Answer from the drawing. Dimensions are ordinates in mm from the lowest x, y and z of the part. A direction names the side the tool comes from. Coordinates: 2 decimals unless noted, no trailing zeros. Order: outer loops, then holes, each group sorted by start corner. A loop starts at its lowest first (then second) coordinate and runs counter-clockwise, first axis right, second up. Notation, with made-up numbers: (54.25, 23) - (79.25, 23) arc R12 cw to (79.25, 43) - close; hole circle Ø2 at (60, 32). An arc over 180 degrees is marked (long way). Answer as a JSON object with one key per item and string values. Group by question number.
1) Section C-C (z = 80.5) is taken. Count the separate pieces of the cut face and the enclosed holes in it, plus the area to 3 significant figures.
2) The mould has two halves that part along X. Classify the marked faces 1, 2 and 3: released by +X, released by -X, zero draft, split by the parting line, or undercut.
3) A tool of negligible diameter and unlimited length cuts with its end or side. For the marked faces 4, 5, 6, 7 and 8, from which of +Z, -Z, +X, -X, +Y, -Y can it reach the whole face along a straight path? Write none if from no direction.
4) Each of these flat-tipped pins is pushed along its axis until it touches: P1, Ø5, axis at x = 74, y = 104.5, coming from the +Z side; P2, Ø5, axis at x = 54, z = 22.5, coming from the +Y side; P3, Ø2, axis at x = 63, z = 83.5, coming from the -Y side; P4, Ø12, axis at x = 94, z = 77.5, coming from the -Y side. Where does it stop, or does it pass through?
5) Section A-A (z = 15) is taken. Give the vertices of the cut face in (x, y) (1 decimal), plus the area to 3 significant figures.
6) Section B-B (y = 87) is taken. Give the vertices of the cut face in (x, z) (1 decimal), plus the area to 3 significant figures.
7) Section D-D (x = 64.5) is taken. Give the vertices of the cut face in (y, z) (1 decimal).
8) Find the intervals of material crossed by line 1 along Z through (x, y) = (31, 68); line 2 along X through (y, z) = (66, 74.5); line 3 along X through (y, z) = (38, 81) (1 decimal), in increasing order.
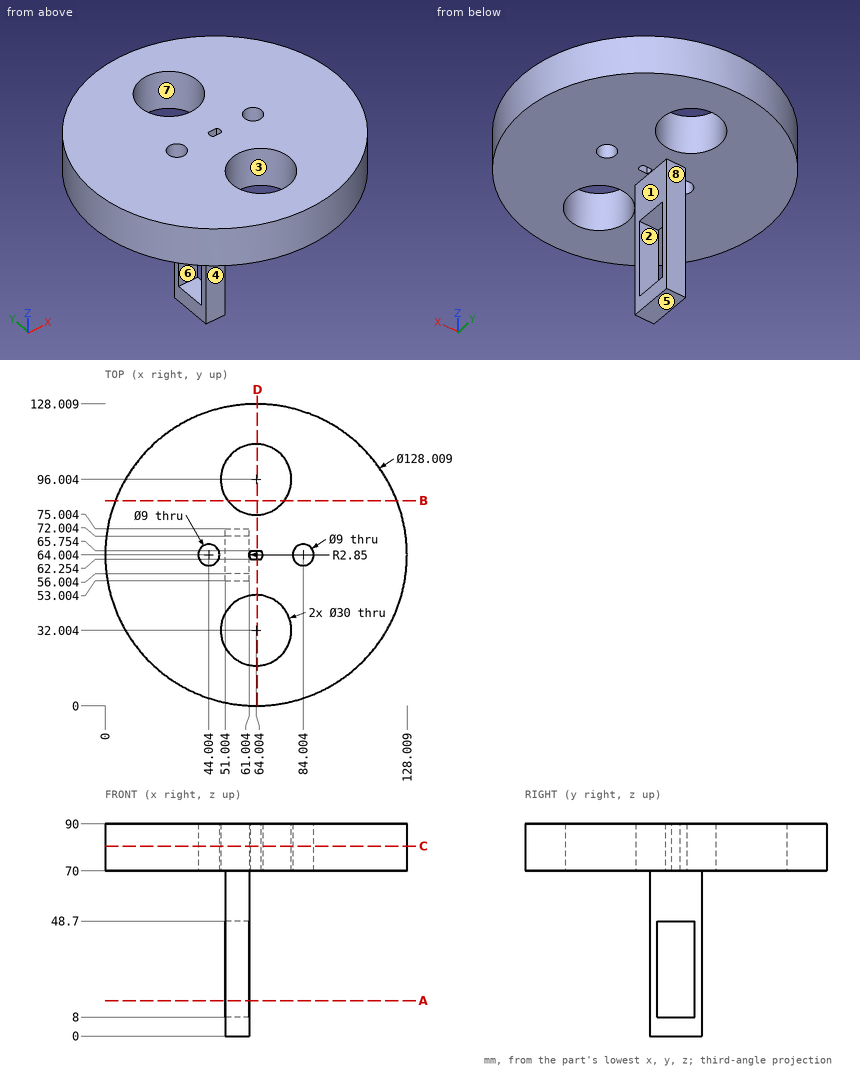
Report:
{
 "1": {"separate pieces": "1", "enclosed holes": "5", "area": "11,300 mm²"},
 "2": {"face 1": "released by +X", "face 2": "zero draft", "face 3": "undercut"},
 "3": {"face 4": "-Z, +X, -X, -Y", "face 5": "-Z, +X, -X, +Y, -Y", "face 6": "+X, -X", "face 7": "+Z, -Z", "face 8": "-Z, +X, -X, +Y"},
 "4": {"P1": "stops at z = 90", "P2": "stops at y = 75", "P3": "stops at y = 0", "P4": "stops at y = 4.67"},
 "5": {"outline": "(51, 53) - (61, 53) - (61, 56) - (51, 56) - close; (51, 72) - (61, 72) - (61, 75) - (51, 75) - close", "area": "60.0 mm²"},
 "6": {"outline": "(4.3, 70) - (52, 70) - (52, 90) - (4.3, 90) - close; (76, 70) - (123.7, 70) - (123.7, 90) - (76, 90) - close", "area": "1,910 mm²"},
 "7": {"outline": "(0, 70) - (17, 70) - (17, 90) - (0, 90) - close; (47, 70) - (62.3, 70) - (62.3, 90) - (47, 90) - close; (65.8, 70) - (81, 70) - (81, 90) - (65.8, 90) - close; (111, 70) - (128, 70) - (128, 90) - (111, 90) - close"},
 "8": {"line 1": "z = 70 to 90", "line 2": "x = 0.03 to 39.97, 48.04 to 79.97, 88.04 to 127.98", "line 3": "x = 5.5 to 50.3, 77.8 to 122.5"}
}
